Input: part model. Units: mm. Frame: model coordinates. Face numbers are marked on the shaded views. Coordinates: 2 decimals unless noted, no trailing zeros. Write each loop counter-clockwise with the first axis right and the second up, starting at its lowest first coordinate (ties: lowest second). Pieces come first, ordered by that corner, then holes.
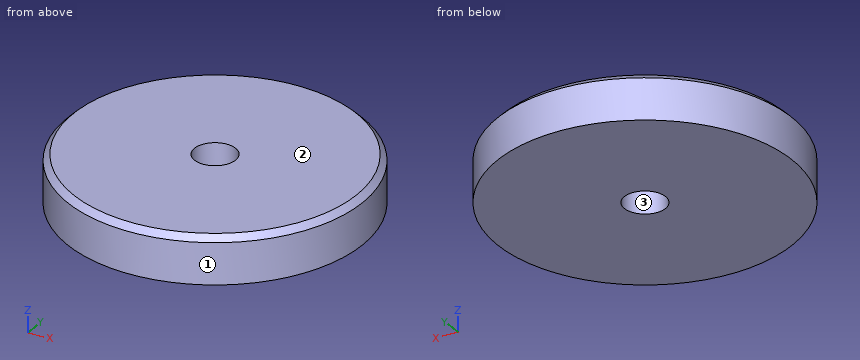
from build123d import *

# Parameters (mm, degrees)
SKETCH1_R           = 12.5
BOSS_EXTRUDE1_DEPTH = 4
CHAMFER1_SIZE       = 0.5
SKETCH7_R           = 1.25
CUT_EXTRUDE1_DEPTH  = 19.12456896
SKETCH10_R          = 1.75
CUT_EXTRUDE2_DEPTH  = 19.12456896


with BuildPart() as part:
    # Sketch1 → Boss-Extrude1 (new body)
    with BuildSketch(Plane.XY):
        Circle(SKETCH1_R)
    extrude(amount=BOSS_EXTRUDE1_DEPTH)

    # Chamfer1
    chamfer1_edges = [part.edges().sort_by_distance(p)[0] for p in [
        (-12.5, 0, 4),
    ]]
    chamfer(chamfer1_edges, length=CHAMFER1_SIZE)

    # Sketch7 → Cut-Extrude1 (cut, through all)
    with BuildSketch(Plane.XY.offset(4)):
        Circle(SKETCH7_R)
    extrude(amount=-CUT_EXTRUDE1_DEPTH, mode=Mode.SUBTRACT)

    # Sketch10 → Cut-Extrude2 (cut, through all)
    with BuildSketch(Plane.XY.offset(4)):
        Circle(SKETCH10_R)
    extrude(amount=-CUT_EXTRUDE2_DEPTH, mode=Mode.SUBTRACT)


solid = part.part
Item 1: Pin query (flat end, axial travel): pin 1 Ø1 at (y, z) = (-1, 1) entering from +X. Return the tip coordinate at first contact, or that it passes through.
Item 2: Material intervals for line 1 (Y direction, x = 0, z = 2.05); line 2 (Y direction, x = 0.75, z = 3.15); line 3 (X direction, y = 1.5, z = 0.3), sorted ascending.
Item 3: Section query C-C, the plane z = 1.25. Return loops of the section in (x, y), then the cut area to 3 significant figures.
Item 4: Section query A-A, the plane x = 0. Return loops of the section in (y, z), then the cut area to 4 significant figures.
Item 5: Pull-direction query (X, two-part tool) for the marked faces 1, 2 and 3; classes: released by +X, released by -X, zero draft, split by the parting line, or undercut.
The answers:
1. pin 1: stops at x = 12.49
2. line 1: y = -12.5 to -1.75, 1.75 to 12.5
2. line 2: y = -12.48 to -1.58, 1.58 to 12.48
2. line 3: x = -12.41 to -0.9, 0.9 to 12.41
3. outline: circle Ø25 at (0, 0); hole circle Ø3.5 at (0, 0)
3. area: 481 mm2
4. outline: (-12.5, 0) - (-1.75, 0) - (-1.75, 4) - (-12, 4) - (-12.5, 3.5) - close; (1.75, 0) - (12.5, 0) - (12.5, 3.5) - (12, 4) - (1.75, 4) - close
4. area: 85.75 mm2
5. face 1: split by the parting line
5. face 2: zero draft
5. face 3: undercut
